```python
from build123d import *

# Parameters (mm, degrees)
F1_DEPTH = 6.2
F2_R     = 13.75
F3_DEPTH = 8.8
F4_R     = 4.5
F4_R_2   = 9
F5_R     = 4.5
F6_DEPTH = 10


with BuildPart() as f1:
    # F0 (on Front) → F1 (new body)
    with BuildSketch(Plane.XZ):
        with BuildLine():
            Line((0, 0), (15, 0))
            ThreePointArc((15, 0), (12.8954858771, 7.662013051), (7.1724741341, 13.1740508119))
            Line((7.1724741341, 13.1740508119), (0, 15))
            Line((0, 15), (-6.6466510201, 13.4470082255))
            ThreePointArc((-6.6466510201, 13.4470082255), (-12.7416593366, 7.9151827111), (-15, 0))
            Line((-15, 0), (0, 0))
        make_face()
        with BuildLine():
            Line((19.3797829829, 0), (15, 0))
            ThreePointArc((15, 0), (12.8954858771, -7.662013051), (7.1724741341, -13.1740508119))
            Line((7.1724741341, -13.1740508119), (27.4034789598, -8.023695977))
            ThreePointArc((27.4034789598, -8.023695977), (21.7298691243, -5.6736098355), (19.3797829829, 0))
        make_face()
        with BuildLine():
            ThreePointArc((7.1724741341, -13.1740508119), (12.8954858771, -7.662013051), (15, 0))
            Line((15, 0), (0, 0))
            Line((0, 0), (-15, 0))
            ThreePointArc((-15, 0), (-12.7416593366, -7.9151827111), (-6.6466510201, -13.4470082255))
            Line((-6.6466510201, -13.4470082255), (0, -15))
            Line((0, -15), (7.1724741341, -13.1740508119))
        make_face()
        with BuildLine():
            ThreePointArc((7.1724741341, 13.1740508119), (12.8954858771, 7.662013051), (15, 0))
            Line((15, 0), (19.3797829829, 0))
            ThreePointArc((19.3797829829, 0), (21.7298691243, 5.6736098355), (27.4034789598, 8.023695977))
            Line((27.4034789598, 8.023695977), (7.1724741341, 13.1740508119))
        make_face()
        with BuildLine():
            Line((0, 15), (7.1724741341, 13.1740508119))
            ThreePointArc((7.1724741341, 13.1740508119), (3.7006241245, 14.5363468963), (0, 15))
        make_face()
        with BuildLine():
            ThreePointArc((0, -15), (3.7006241245, -14.5363468963), (7.1724741341, -13.1740508119))
            Line((7.1724741341, -13.1740508119), (0, -15))
        make_face()
        with BuildLine():
            ThreePointArc((27.4034789598, 8.023695977), (21.7298691243, 5.6736098355), (19.3797829829, 0))
            ThreePointArc((19.3797829829, 0), (21.7298691243, -5.6736098355), (27.4034789598, -8.023695977))
            ThreePointArc((27.4034789598, -8.023695977), (33.0770887953, -5.6736098355), (35.4271749368, 0))
            ThreePointArc((35.4271749368, 0), (33.0770887953, 5.6736098355), (27.4034789598, 8.023695977))
        make_face()
        with BuildLine():
            Line((-6.6466510201, 13.4470082255), (0, 15))
            ThreePointArc((0, 15), (-3.4128343512, 14.6065930898), (-6.6466510201, 13.4470082255))
        make_face()
        with BuildLine():
            ThreePointArc((-6.6466510201, -13.4470082255), (-3.4128343512, -14.6065930898), (0, -15))
            Line((0, -15), (-6.6466510201, -13.4470082255))
        make_face()
        with BuildLine():
            Line((-18.8063090901, 0), (-15, 0))
            ThreePointArc((-15, 0), (-12.7416593366, 7.9151827111), (-6.6466510201, 13.4470082255))
            Line((-6.6466510201, 13.4470082255), (-27.4034789598, 8.5971698697))
            ThreePointArc((-27.4034789598, 8.5971698697), (-21.3243618459, 6.0791171139), (-18.8063090901, 0))
        make_face()
        with BuildLine():
            ThreePointArc((-6.6466510201, -13.4470082255), (-12.7416593366, -7.9151827111), (-15, 0))
            Line((-15, 0), (-18.8063090901, 0))
            ThreePointArc((-18.8063090901, 0), (-21.3243618459, -6.0791171139), (-27.4034789598, -8.5971698697))
            Line((-27.4034789598, -8.5971698697), (-6.6466510201, -13.4470082255))
        make_face()
        with BuildLine():
            ThreePointArc((-27.4034789598, -8.5971698697), (-21.3243618459, -6.0791171139), (-18.8063090901, 0))
            ThreePointArc((-18.8063090901, 0), (-21.3243618459, 6.0791171139), (-27.4034789598, 8.5971698697))
            ThreePointArc((-27.4034789598, 8.5971698697), (-36.0006488296, 0), (-27.4034789598, -8.5971698697))
        make_face()
    extrude(amount=F1_DEPTH)

    # F2 (on face) → F3 (join)
    with BuildSketch(Plane(origin=(0, 0, 0), x_dir=(-1, 0, 0), z_dir=(0, 1, 0))):
        Circle(F2_R)
    extrude(amount=F3_DEPTH)

    # F4 (on face) + F5 (on face) → F6 (cut)
    with BuildSketch(Plane.XZ.offset(6.2)):
        with Locations((27.4034789598, 0)):
            Circle(F4_R)
        Circle(F4_R_2)
    with BuildSketch(Plane.XZ.offset(6.2)):
        with Locations((-27.4034789598, 0)):
            Circle(F5_R)
    extrude(amount=-F6_DEPTH, mode=Mode.SUBTRACT)


solid = f1.part
```
For this review, take the finished solid that the model builds, in its own axes (mm). A direction names the side the tool comes from. Coordinates: 2 decimals unless noted, no trailing zeros. Order: outer loops, then holes, each group sorted by start corner. A loop starts at its lowest first (then second) coordinate and runs counter-clockwise, first axis right, second up. Notation, with made-up numbers: (75, -2) - (96, -2) arc R18 ccw to (96, 4) - close; hole circle Ø9 at (89, 77). An arc over 180 degrees is marked (long way). Answer as a JSON object with one key per item and string values. Group by question number.
1. For probe 1 along X at (y, z) = (-5.5, 4); probe 2 along X at (y, z) = (-4, -1); probe 3 along Y at (x, z) = (-2.5, -8), list the stretches that pass through material, from the lowest coordinate up.
2. The part is to be moulded in two halves that separate along X. For faces 1 (the flat face through (-9, -6.2, -3)), 2 (the cylindrical face through (-1.172, -1.27, 8.923)), 3 (the cylindrical face through (2.981, 4.338, -13.423)), say which applies: pulls with the +X half, pulls with the -X half, needs draft (parallel to the pull), parting line crosses it, or undercut.
3. Clearance check with flat-ended pins moving along their axes: P1, Ø1, axis at y = 2.5, z = -7.5, coming from the +X side; P2, Ø1.5, axis at x = -13.5, y = 5.5, coming from the +Z side; P3, Ø9, axis at x = 3.5, z = 0.5, coming from the -Y side. State where each tip first meets the part, or that it passes through.
4. For faces 4 (the flat face through (17.43, -3.057, 10.563)), 5 (the flat face through (0, 3.8, 0)), list the 3-axis set-ups (+Z, -Z, +X, -X, +Y, -Y) from which the entire face can be reached by the end or side of a thin tool; tool diameter is ignored.
5. We need section C-C on z = -12.5. State the section outline as (x, y) points, then the cut area to 3 significant figures.
6. We need section B-B on z = -2. State the section outline as (x, y) points, then the cut area to 3 significant figures.
7. We need section D-D on y = 5.25. State the section outline as (x, z) points, then the cut area to 3 significant figures.
8. We need section A-A on y = -2.5. State the section outline as (x, z) points, then the cut area to 3 significant figures.
Final values:
{
 "1": {"probe 1": "-35.01 to -29.47, -25.34 to -8.06, 8.06 to 25.34, 29.47 to 34.36", "probe 2": "-35.94 to -31.79, -23.02 to -8.94, 8.94 to 23.02, 31.79 to 35.36", "probe 3": "3.8 to 8.8"},
 "2": {"face 1": "needs draft", "face 2": "undercut", "face 3": "parting line crosses it"},
 "3": {"P1": "x = 11.83", "P2": "z = 5.15", "P3": "y = 3.8"},
 "4": {"face 4": "+Z, +X, +Y, -Y", "face 5": "-Y"},
 "5": {"outline": "(-10.7, -6.2) - (9.82, -6.2) - (9.82, 0) - (5.73, 0) - (5.73, 8.8) - (-5.73, 8.8) - (-5.73, 0) - (-10.7, 0) - close", "area": "228 mm²"},
 "6": {"outline": "(-35.76, -6.2) - (-31.43, -6.2) - (-31.43, 0) - (-35.76, 0) - close; (-23.37, -6.2) - (-8.77, -6.2) - (-8.77, 3.8) - (8.77, 3.8) - (8.77, -6.2) - (23.37, -6.2) - (23.37, 0) - (13.6, 0) - (13.6, 8.8) - (-13.6, 8.8) - (-13.6, 0) - (-23.37, 0) - close; (31.43, -6.2) - (35.17, -6.2) - (35.17, 0) - (31.43, 0) - close", "area": "404 mm²"},
 "7": {"outline": "circle Ø27.5 at (0, 0)", "area": "594 mm²"},
 "8": {"outline": "(-27.4, -8.6) - (-6.65, -13.45) arc R15 ccw to (7.17, -13.17) - (27.4, -8.02) arc R8.02 ccw to (27.4, 8.02) - (7.17, 13.17) arc R15 ccw to (-6.65, 13.45) - (-27.4, 8.6) arc R8.6 ccw to start; hole circle Ø9 at (-27.4, 0); hole circle Ø18 at (0, 0); hole circle Ø9 at (27.4, 0)", "area": "1,120 mm²"}
}
